```python
from build123d import *

# Parameters (mm, degrees)
F0_R     = 1.5
F1_DEPTH = 6.2
F2_R     = 1.5
F3_R     = 2
F4_DEPTH = 7.5


with BuildPart() as f1:
    # F0 (on Front) → F1 (new body)
    with BuildSketch(Plane.XZ):
        with BuildLine():
            Line((-12, 0), (0, 0))
            Line((0, 0), (0, 10))
            Line((0, 10), (-12, 10))
            ThreePointArc((-12, 10), (-12.585786, 8.585786), (-14, 8))
            Line((-14, 8), (-14, 2))
            ThreePointArc((-14, 2), (-12.585786, 1.414214), (-12, 0))
        make_face()
        with Locations((-3.5, 5)):
            Circle(F0_R, mode=Mode.SUBTRACT)
    extrude(amount=F1_DEPTH)

    # F2
    f2_edges = [f1.edges().sort_by_distance(p)[0] for p in [
        (-6, -6.2, 10),
        (-6, 0, 10),
        (-6, 0, 0),
        (-6, -6.2, 0),
    ]]
    fillet(f2_edges, radius=F2_R)

    # F3 (on face) → F4 (cut)
    with BuildSketch(Plane(origin=(-14, 0, 0), x_dir=(0, -1, 0), z_dir=(-1, 0, 0))):
        with Locations((3.1, 5)):
            Circle(F3_R)
    extrude(amount=-F4_DEPTH, mode=Mode.SUBTRACT)


solid = f1.part
```
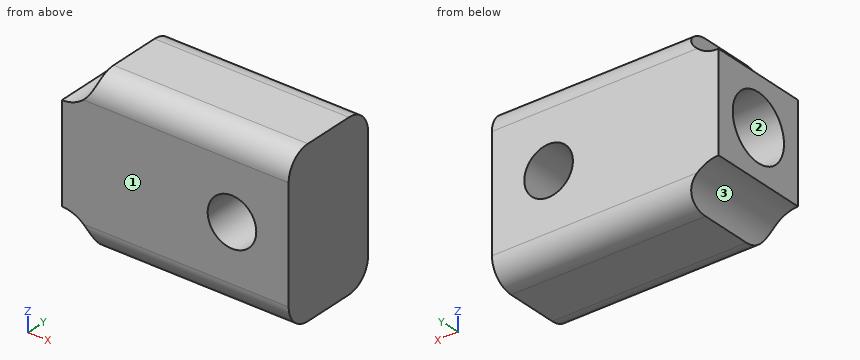
Design review of the part built by this model. Coordinates are the model's own, in mm. Face numbers are marked on the shaded views. Coordinates: 2 decimals unless noted, no trailing zeros. Loops run counter-clockwise (first coordinate to the right, second up) from the corner with the lowest first, then second, coordinate; pieces in that order, holes last. Notation, with made-up numbers: (-36, 89) -> (3, 89) arc R12 cw to (3, 107) -> close; hole circle Ø4 at (26, 52.5). An arc over 180 degrees is marked (long way). Answer as a JSON object with one key per item and string values.
Q1. Clearance check with a flat-ended pin moving along its axis: pin 1 Ø3 at (x, y) = (-8.5, -5.5) entering from +Z. State where the tip first meets the part, or that it passes through.
Answer block:
{"pin 1": "stops at z = 10"}
Q2. Take a section at A-A on z = 5. Give the boundary of the cut face in (x, y), plus the area to 3 significant figures.
Answer block:
{"outline": "(-14, -6.2) -> (-5, -6.2) -> (-5, 0) -> (-14, 0) -> (-14, -1.1) -> (-6.5, -1.1) -> (-6.5, -5.1) -> (-14, -5.1) -> close; (-2, -6.2) -> (0, -6.2) -> (0, 0) -> (-2, 0) -> close", "area": "38.2 mm^2"}
Q3. Take a section at B-B on x = -10.75. Give the boundary of the cut face in (y, z), plus the area to 3 significant figures.
Answer block:
{"outline": "(-6.2, 1.5) arc R1.5 ccw to (-4.7, 0) -> (-1.5, 0) arc R1.5 ccw to (0, 1.5) -> (0, 8.5) arc R1.5 ccw to (-1.5, 10) -> (-4.7, 10) arc R1.5 ccw to (-6.2, 8.5) -> close; hole circle Ø4 at (-3.1, 5)", "area": "47.5 mm^2"}
Q4. Take a section at C-C on y = -3.1. Give the boundary of the cut face in (x, z), plus the area to 3 significant figures.
Answer block:
{"outline": "(-14, 2) arc R2 cw to (-12, 0) -> (0, 0) -> (0, 10) -> (-12, 10) arc R2 cw to (-14, 8) -> (-14, 7) -> (-6.5, 7) -> (-6.5, 3) -> (-14, 3) -> close; hole circle Ø3 at (-3.5, 5)", "area": "96.6 mm^2"}
Q5. Take a section at D-D on x = -3.5. Give the boundary of the cut face in (y, z).
Answer block:
{"outline": "(-6.2, 1.5) arc R1.5 ccw to (-4.7, 0) -> (-1.5, 0) arc R1.5 ccw to (0, 1.5) -> (0, 3.5) -> (-6.2, 3.5) -> close; (-6.2, 6.5) -> (0, 6.5) -> (0, 8.5) arc R1.5 ccw to (-1.5, 10) -> (-4.7, 10) arc R1.5 ccw to (-6.2, 8.5) -> close"}
Q6. The part is to be moulded in two halves that separate along Z. For the marked faces 1, 2 and 3, say which applies: +Z half, -Z half, draft (parallel to the pull), parting line (faces both ways), or undercut.
Answer block:
{"face 1": "draft", "face 2": "undercut", "face 3": "-Z half"}
Q7. To check wall thickness, follow L1, parallel to Z at x = -3.5, y = -4.25; L2, parallel to Z at x = -10, y = -3.1; L3, parallel to X at y = -3.75, z = 5.5. State the ranges of each line that lie inside material, in increasing order.
Answer block:
{"L1": "z = 0 to 3.5, 6.5 to 10", "L2": "z = 0 to 3, 7 to 10", "L3": "x = -6.5 to -4.91, -2.09 to 0"}
